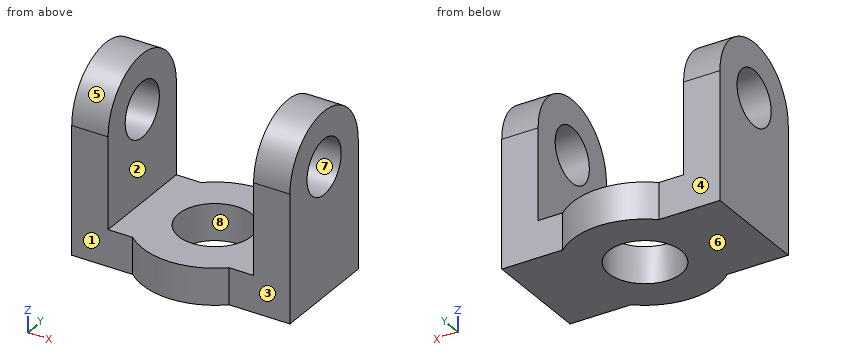
```python
from build123d import *

# Parameters (mm, degrees)
F0_R     = 10
F1_DEPTH = 10
F2_DEPTH = 50
F3_R     = 7.5
F4_DEPTH = 60.001


with BuildPart() as f1:
    # F0 (on Top) → F1 (new body)
    with BuildSketch(Plane.XY):
        Polygon((0, 30), (0, 0), (10, 0), (10, 15), (10, 30), align=None)
        with BuildLine():
            Line((10, 15), (10, 0))
            Line((10, 0), (16.7712434447, 0))
            ThreePointArc((16.7712434447, 0), (11.7712434447, 6.7712434447), (10, 15))
        make_face()
        with BuildLine():
            ThreePointArc((10, 15), (11.7712434447, 6.7712434447), (16.7712434447, 0))
            Line((16.7712434447, 0), (43.2287565553, 0))
            ThreePointArc((43.2287565553, 0), (48.2287565553, 6.7712434447), (50, 15))
            ThreePointArc((50, 15), (48.2287565553, 23.2287565553), (43.2287565553, 30))
            Line((43.2287565553, 30), (16.7712434447, 30))
            ThreePointArc((16.7712434447, 30), (11.7712434447, 23.2287565553), (10, 15))
        make_face()
        with Locations((30, 15)):
            Circle(F0_R, mode=Mode.SUBTRACT)
        with BuildLine():
            Line((43.2287565553, 0), (16.7712434447, 0))
            ThreePointArc((16.7712434447, 0), (30, -5), (43.2287565553, 0))
        make_face()
        with BuildLine():
            Line((10, 30), (10, 15))
            ThreePointArc((10, 15), (11.7712434447, 23.2287565553), (16.7712434447, 30))
            Line((16.7712434447, 30), (10, 30))
        make_face()
        with BuildLine():
            ThreePointArc((50, 15), (48.2287565553, 6.7712434447), (43.2287565553, 0))
            Line((43.2287565553, 0), (50, 0))
            Line((50, 0), (50, 15))
        make_face()
        with BuildLine():
            ThreePointArc((43.2287565553, 30), (30, 35), (16.7712434447, 30))
            Line((16.7712434447, 30), (43.2287565553, 30))
        make_face()
        Polygon((50, 15), (50, 0), (60, 0), (60, 30), (50, 30), align=None)
        with BuildLine():
            ThreePointArc((43.2287565553, 30), (48.2287565553, 23.2287565553), (50, 15))
            Line((50, 15), (50, 30))
            Line((50, 30), (43.2287565553, 30))
        make_face()
    extrude(amount=F1_DEPTH)

    # F0 (on Top) → F2 (join)
    with BuildSketch(Plane.XY):
        Polygon((0, 30), (0, 0), (10, 0), (10, 15), (10, 30), align=None)
        Polygon((50, 15), (50, 0), (60, 0), (60, 30), (50, 30), align=None)
    extrude(amount=F2_DEPTH)

    # F3 (on face) → F4 (cut, through all)
    with BuildSketch(Plane(origin=(0, 0, 0), x_dir=(0, -1, 0), z_dir=(-1, 0, 0))):
        with Locations((-15, 35)):
            Circle(F3_R)
        with BuildLine():
            Line((-30, 50), (-30, 35))
            ThreePointArc((-30, 35), (-25.6066017178, 45.6066017178), (-15, 50))
            Line((-15, 50), (-30, 50))
        make_face()
        with BuildLine():
            Line((0, 50), (-15, 50))
            ThreePointArc((-15, 50), (-4.3933982822, 45.6066017178), (0, 35))
            Line((0, 35), (0, 50))
        make_face()
    extrude(amount=-F4_DEPTH, mode=Mode.SUBTRACT)


solid = f1.part
```
Could you check a few things on this model? Use its own coordinates, in mm. Face numbers are marked on the shaded views. A direction names the side the tool comes from. Round coordinates to 2 decimals unless told otherwise and drop trailing zeros. Write each loop counter-clockwise with the first axis right and the second up, starting at its lowest first coordinate (ties: lowest second). Pieces come first, ordered by that corner, then holes.
(1) Suppose I cut it at C-C on z = 12.5. Write out the boundary of the cut face in (x, y), and give its area (3 significant figures).
Findings below:
outline: (0, 0) - (10, 0) - (10, 30) - (0, 30) - close; (50, 0) - (60, 0) - (60, 30) - (50, 30) - close
area: 600 mm2
(2) Thinking about a two-plate mould opening in Y: for the marked faces 5, 6, 7 and 8, which applies, +Y half, -Y half, draft (parallel to the pull), parting line (faces both ways), or undercut?
Findings below:
face 5: parting line
face 6: draft
face 7: undercut
face 8: undercut
(3) Suppose I cut it at D-D on y = 16. Write out the boundary of the cut face in (x, z).
Findings below:
outline: (0, 0) - (20.05, 0) - (20.05, 10) - (10, 10) - (10, 27.57) - (0, 27.57) - close; (0, 42.43) - (10, 42.43) - (10, 49.97) - (0, 49.97) - close; (39.95, 0) - (60, 0) - (60, 27.57) - (50, 27.57) - (50, 10) - (39.95, 10) - close; (50, 42.43) - (60, 42.43) - (60, 49.97) - (50, 49.97) - close
(4) Which directions (+Z, -Z, +X, -X, +Y, -Y) give clear straight access to the entire face, cutting with the end or side of a thin tool? Please do the marked faces 1, 2, 3 and 4.
Findings below:
face 1: +Z, -Z, -X, -Y
face 2: +Z, +Y, -Y
face 3: +Z, -Z, +X, -Y
face 4: +Z, -Z, -X, +Y
(5) If I drill on probe 1 along Z at (x, y) = (4, 15); probe 2 along X at (y, z) = (8, 23); probe 3 along Y at (x, z) = (30, 7.5), over which ranges is the centre line in solid material (lowest first)?
Findings below:
probe 1: z = 0 to 27.5, 42.5 to 50
probe 2: x = 0 to 10, 50 to 60
probe 3: y = -5 to 5, 25 to 35
(6) Suppose I cut it at B-B on x = 30. Write out the boundary of the cut face in (y, z).
Findings below:
outline: (-5, 0) - (5, 0) - (5, 10) - (-5, 10) - close; (25, 0) - (35, 0) - (35, 10) - (25, 10) - close
(7) Suppose I cut it at A-A on z = 29. Write out the boundary of the cut face in (x, y), and give its area (3 significant figures).
Findings below:
outline: (0, 0) - (10, 0) - (10, 10.5) - (0, 10.5) - close; (0, 19.5) - (10, 19.5) - (10, 30) - (0, 30) - close; (50, 0) - (60, 0) - (60, 10.5) - (50, 10.5) - close; (50, 19.5) - (60, 19.5) - (60, 30) - (50, 30) - close
area: 420 mm2
(8) For pin 1 (1.5 mm diameter, centred on x = 18, y = 29.5, fed in from +Z); pin 2 (18.5 mm diameter, centred on x = 8.5, z = 23.5, fed in from -Y); pin 3 (12 mm diameter, centred on x = 52, y = 5, fed in from +Z), each with a flat end and sliding along its axis, tell me the tip position at first contact or that it passes through.
Findings below:
pin 1: stops at z = 10
pin 2: stops at y = 0
pin 3: stops at z = 49.46
